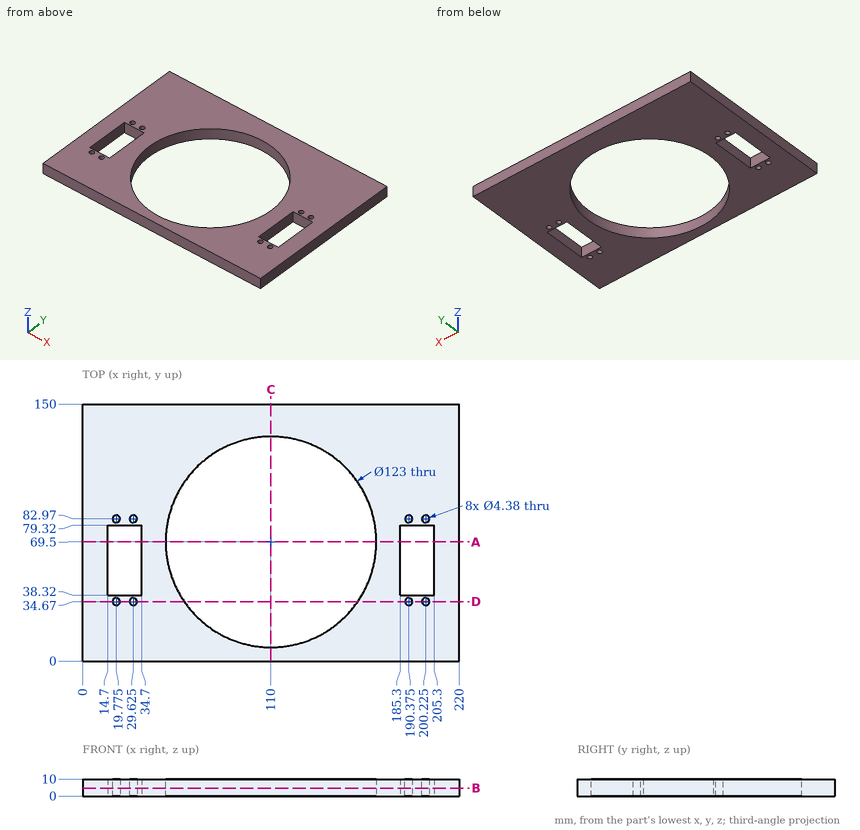
The figure shows three views and two pictorial views of one solid part (mm, origin at its lowest corner). Answer the questions. Coordinates: 2 decimals unless noted, no trailing zeros. Write each loop counter-clockwise with the first axis right and the second up, starting at its lowest first coordinate (ties: lowest second). Pieces come first, ordered by that corner, then holes. Notation, with made-up numbers: (18, 12) -> (50, 12) arc R25 ccw to (50, 37) -> close; hole circle Ø6 at (29, 11.25). An arc over 180 degrees is marked (long way). Return JSON: item names as keys, results as strings.
(1) The part is cut by section D-D on y = 34.67. Give the vertices of the cut face in (x, z) (1 decimal), then the cut area to 3 significant figures.
Answers below:
{"outline": "(0, 0) -> (17.6, 0) -> (17.6, 10) -> (0, 10) -> close; (22, 0) -> (27.4, 0) -> (27.4, 10) -> (22, 10) -> close; (31.8, 0) -> (59.3, 0) -> (59.3, 10) -> (31.8, 10) -> close; (160.7, 0) -> (188.2, 0) -> (188.2, 10) -> (160.7, 10) -> close; (192.6, 0) -> (198, 0) -> (198, 10) -> (192.6, 10) -> close; (202.4, 0) -> (220, 0) -> (220, 10) -> (202.4, 10) -> close", "area": "1,010 mm^2"}
(2) The part is cut by section C-C on x = 110. Give the vertices of the cut face in (y, z), then the cut area to 3 significant figures.
Answers below:
{"outline": "(0, 0) -> (8, 0) -> (8, 10) -> (0, 10) -> close; (131, 0) -> (150, 0) -> (150, 10) -> (131, 10) -> close", "area": "270 mm^2"}
(3) The part is cut by section A-A on y = 69.5. Give the vertices of the cut face in (x, z), then the cut area to 3 significant figures.
Answers below:
{"outline": "(0, 0) -> (14.7, 0) -> (14.7, 10) -> (0, 10) -> close; (34.7, 0) -> (48.5, 0) -> (48.5, 10) -> (34.7, 10) -> close; (171.5, 0) -> (185.3, 0) -> (185.3, 10) -> (171.5, 10) -> close; (205.3, 0) -> (220, 0) -> (220, 10) -> (205.3, 10) -> close", "area": "570 mm^2"}
(4) Each of these flat-tipped pins is pushed along its axis until it touches: P1, Ø2.5, axis at x = 190.375, y = 34.67, coming from the -Z side; P2, Ø3, axis at x = 27.5, y = 79.5, coming from the -Z side. Where does it stop, or does it pass through?
Answers below:
{"P1": "through", "P2": "z = 0"}
(5) The part is cut by section B-B on z = 4.75. State how many separate pieces and enclosed holes the cut face has, then the cut area to 3 significant figures.
Answers below:
{"separate pieces": "1", "enclosed holes": "11", "area": "19,400 mm^2"}
(6) Consider line 1 along Y through (x, z) = (23, 1.75); line 2 along X through (y, z) = (33, 8.5); line 3 along X through (y, z) = (84, 7.25). Determine where each line is inside the solid, lowest interval first. Write a range as from..to.
Answers below:
{"line 1": "0..38.32, 79.32..150", "line 2": "0..18.36, 21.19..28.21, 31.04..60.5, 159.5..188.96, 191.79..198.81, 201.64..220", "line 3": "0..17.84, 21.71..27.69, 31.56..50.23, 169.77..188.44, 192.31..198.29, 202.16..220"}
